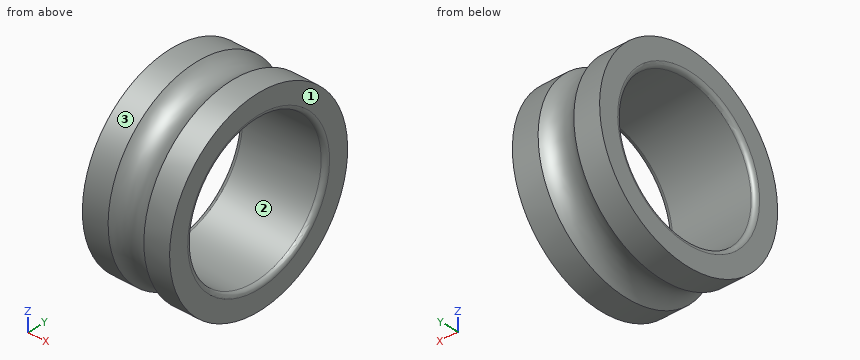
```python
from build123d import *


with BuildPart() as part:
    # Esquisse1 → Base-R_volution (revolve)
    with BuildSketch(Plane(origin=(0, 0, 0), x_dir=(1, 0, 0), z_dir=(0, 1, 0)), mode=Mode.PRIVATE) as base_r_volution_sk:
        with BuildLine():
            Line((0, 13.3), (0, 10.6))
            ThreePointArc((0, 10.6), (0.175735931, 10.175735931), (0.6, 10))
            Line((0.6, 10), (11.4, 10))
            ThreePointArc((11.4, 10), (11.824264069, 10.175735931), (12, 10.6))
            Line((12, 10.6), (12, 13.3))
            Line((12, 13.3), (8.459674775, 13.3))
            ThreePointArc((8.459674775, 13.3), (6, 12.2), (3.540325225, 13.3))
            Line((3.540325225, 13.3), (0, 13.3))
        make_face()
    revolve(base_r_volution_sk.sketch.rotate(Axis((0, 0, 0), (1, 0, 0)), 180), axis=Axis((0, 0, 0), (1, 0, 0)))


solid = part.part
```
Read the model definition and answer for the solid it produces. Units are mm, in the model's axes. Face numbers are marked on the shaded views. Give positions to 0.01 mm unless a question says otherwise; leave off trailing zeros. Write each loop counter-clockwise with the first axis right and the second up, starting at its lowest first coordinate (ties: lowest second). Pieces come first, ordered by that corner, then holes. Notation, with made-up numbers: (46, 0.25) - (102, 0.25) arc R17 ccw to (102, 14.25) - close; hole circle Ø6 at (53, 52). An arc over 180 degrees is marked (long way). Write item = value, one per line. Start each with the question number.
Item 1: Each of these flat-tipped pins is pushed along its axis until it touches: P1, Ø2, axis at x = 3.5, z = 4, coming from the +Y side; P2, Ø3, axis at x = 6, z = 10.5, coming from the +Y side; P3, Ø2, axis at x = 7, z = -7.5, coming from the +Y side. Where does it stop, or does it pass through?
Item 2: Find section C-C (x = 9.5). Give the vertices of the cut face in (y, z).
Item 3: Find the intervals of material crossed by probe 1 along Y at (x, z) = (3, 0); probe 2 along Z at (x, y) = (5.5, 0.5); probe 3 along Z at (x, y) = (3.25, -8.5), in increasing order. Write a range as [from, to].
Item 4: Find section A-A (y = 0). Give the vertices of the cut face in (x, z).
Item 5: The mould has two halves that part along Z. Classify the marked faces 1, 2 and 3: +Z half, -Z half, draft (parallel to the pull), parting line (faces both ways), or undercut.
Item 6: Find section D-D (x = 7). Give the vertices of the cut face in (y, z), then the cut area to 3 significant figures.
Response:
q1.P1 = 12.96
q1.P2 = 8.24
q1.P3 = 10.7
q2.outline = circle Ø26.6 at (0, 0); hole circle Ø20 at (0, 0)
q3.probe_1 = [-13.3, -10], [10, 13.3]
q3.probe_2 = [-12.23, -9.99], [9.99, 12.23]
q3.probe_3 = [-10.23, -5.27], [5.27, 10.23]
q4.outline = (0, -13.3) - (3.54, -13.3) arc R3.3 cw to (8.46, -13.3) - (12, -13.3) - (12, -10.6) arc R0.6 ccw to (11.4, -10) - (0.6, -10) arc R0.6 ccw to (0, -10.6) - close; (0, 10.6) arc R0.6 ccw to (0.6, 10) - (11.4, 10) arc R0.6 ccw to (12, 10.6) - (12, 13.3) - (8.46, 13.3) arc R3.3 cw to (3.54, 13.3) - (0, 13.3) - close
q5.face_1 = draft
q5.face_2 = undercut
q5.face_3 = parting line
q6.outline = circle Ø24.71 at (0, 0); hole circle Ø20 at (0, 0)
q6.area = 165 mm²
